Print and shaded views of the part. All mm, measured from the part's lowest x, y and z. A direction names the side the tool comes from. Give positions to 0.01 mm unless a question says otherwise; leave off trailing zeros. Loops run counter-clockwise (first coordinate to the right, second up) from the corner with the lowest first, then second, coordinate; pieces in that order, holes last. Notation, with made-up numbers: M 10,35 L 44,35 A15 cw 44,57 Z; hole C 50,28 d7. An arc over 180 degrees is marked long. Answer as CSV lines item,"result".
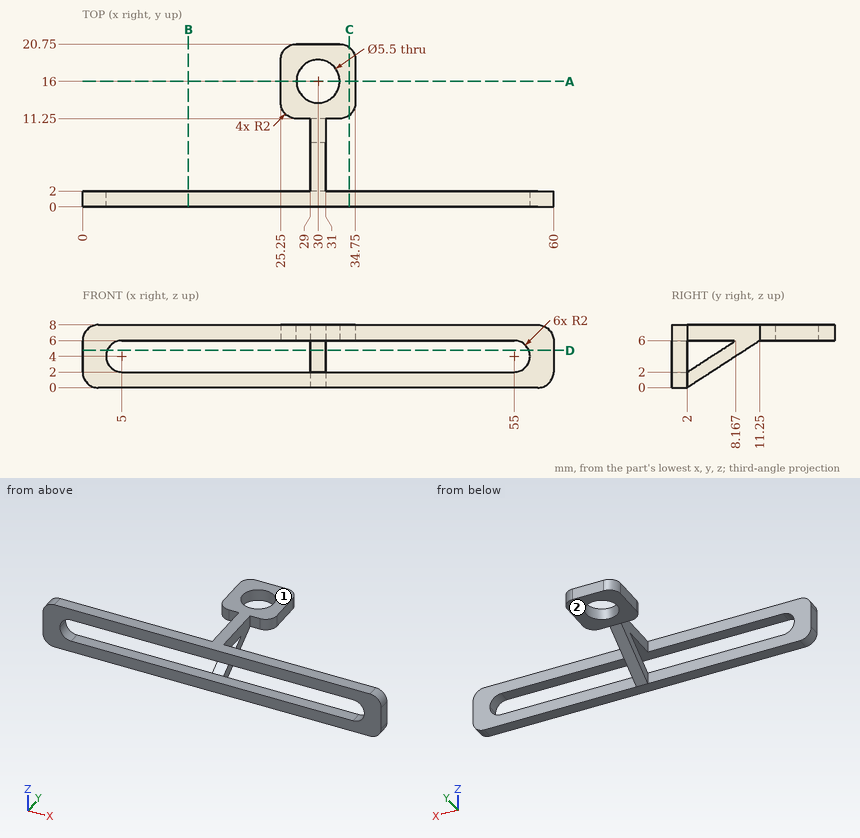
Q1. Cut at B-B (x = 13.5). Write the cut outline in (y, z).
Solution:
outline,"M 0,0 L 2,0 L 2,2 L 0,2 Z; M 0,6 L 2,6 L 2,8 L 0,8 Z"
Q2. Cut at C-C (x = 34). Write the cut outline in (y, z).
Solution:
outline,"M 0,0 L 2,0 L 2,2 L 0,2 Z; M 0,6 L 2,6 L 2,8 L 0,8 Z; M 11.69,6 L 20.31,6 L 20.31,8 L 11.69,8 Z"
Q3. Cut at D-D (z = 4.75). Write the cut outline in (x, y).
Solution:
outline,"M 0,0 L 3.15,0 L 3.15,2 L 0,2 Z; M 29,6.24 L 31,6.24 L 31,9.32 L 29,9.32 Z; M 56.85,0 L 60,0 L 60,2 L 56.85,2 Z"
Q4. Wall check: line 1 (Y direction, x = 30, z = 7.35); line 2 (Y direction, x = 8, z = 6.25); line 3 (Z direction, x = 33.5, y = 15.75). Give the ranges that are in metal, low to high. Write a range as [from, to].
Solution:
line 1,"y = [0, 13.25], [18.75, 20.75]"
line 2,"y = [0, 2]"
line 3,"z = [6, 8]"
Q5. Cut at A-A (y = 16). Write the cut outline in (x, z).
Solution:
outline,"M 25.25,6 L 27.25,6 L 27.25,8 L 25.25,8 Z; M 32.75,6 L 34.75,6 L 34.75,8 L 32.75,8 Z"
Q6. Which spindle directions (+Z, -Z, +X, -X, +Y, -Y) get a long thin tool onto all of the face, cutting with end or side? Do the marked faces 1 and 2. Say none if no direction does.
Solution:
face 1,"+Z, +X, -X, +Y, -Y"
face 2,"-Z, +X, -X, +Y"
Q7. Pin check, flat tips, straight feed: P1, Ø2.5, axis at y = 5, z = 3.5, coming from the +X side; P2, Ø1, axis at y = 15.5, z = 7, coming from the -X side; P3, Ø0.6, axis at y = 16, z = 6.5, coming from the +X side. Stop position of each tip, or through.
Solution:
P1,"stops at x = 31"
P2,"stops at x = 25.25"
P3,"stops at x = 34.75"
